Geometry check sheet. Reference: drawing and pictorial views, mm from the part's lowest x, y, z. Give positions to 0.01 mm unless a question says otherwise; leave off trailing zeros.
Item 1: Release check for a two-part mould opening along X. For the marked faces 1, 2 and 3 record: released by +X, released by -X, zero draft, split by the parting line, or undercut.
Item 2: Sectioned sample at A-A on y = 15.5. Count the separate pieces of the cut face and the enclosed holes in it, and give its area (3 significant figures).
Item 3: Material ranges on line 1 along Z through (x, y) = (30, 7.5) (1 decimal); line 2 along Z through (x, y) = (17, 33) (1 decimal); line 3 along X through (y, z) = (25, 39.5), recorded low to high.
Item 4: Gauge pin test, flat ends, axial feed: P1, Ø2, axis at y = 52, z = 51.5, coming from the -X side; P2, Ø10, axis at x = 49.5, y = 34, coming from the -Z side; P3, Ø4, axis at x = 51, y = 55.5, coming from the -Z side (1 decimal); P4, Ø5.5, axis at x = 28.92, z = 46.72, coming from the +Y side. Record the tip position at first contact, or that the pin passes through.
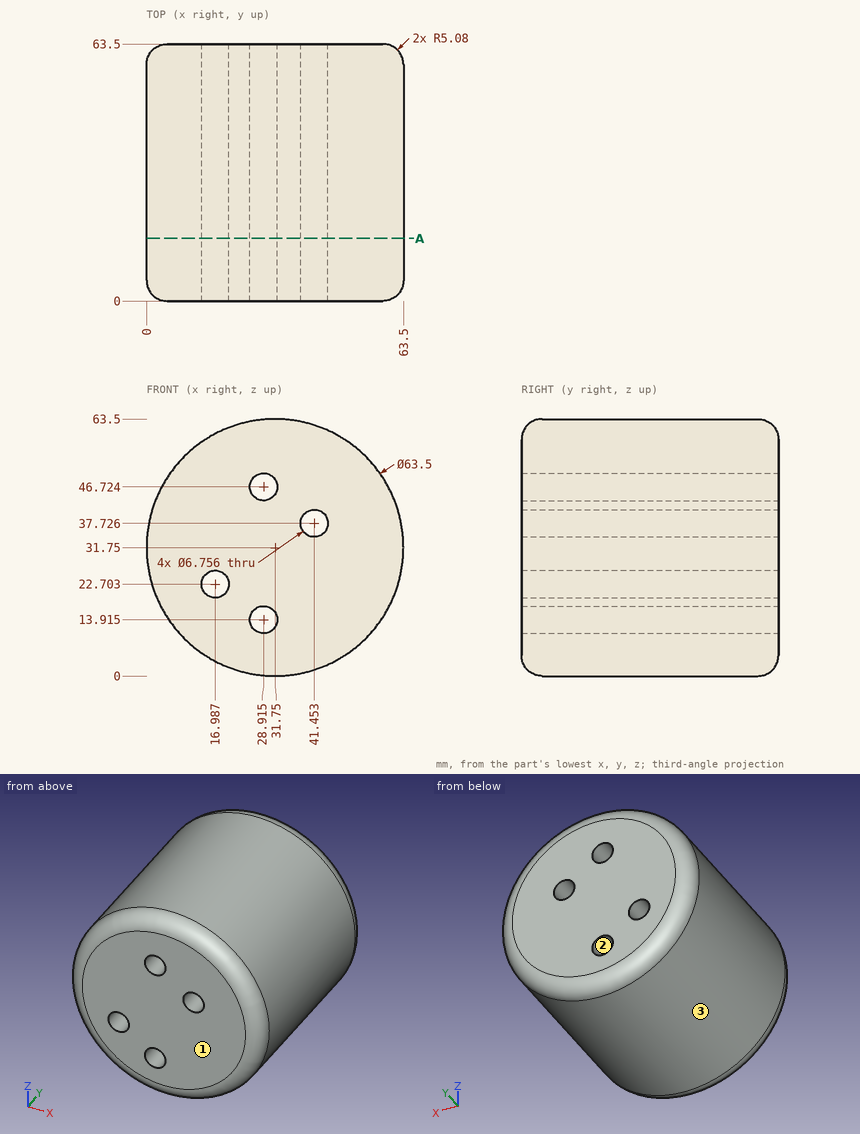
Report:
1. face 1: zero draft
1. face 2: undercut
1. face 3: split by the parting line
2. separate pieces: 1
2. enclosed holes: 4
2. area: 3,020 mm2
3. line 1: z = 0 to 10.7, 17.1 to 43.5, 49.9 to 63.5
3. line 2: z = 3.6 to 19.3, 26.1 to 59.9
3. line 3: x = 0.96 to 38.58, 44.33 to 62.54
4. P1: stops at x = 6.13
4. P2: stops at z = 2.67
4. P3: stops at z = 5.1
4. P4: passes through
